```python
from build123d import *

# Parameters (mm, degrees)
F0_R     = 15.920661
F1_DEPTH = 25.4
F2_DEPTH = 65.786
F3_DEPTH = 76.2
F4_DEPTH = 61.214


with BuildPart() as f1:
    # F0 (on Top) → F1 (new body)
    with BuildSketch(Plane.XY):
        with Locations((46.579406, 0)):
            Circle(F0_R)
        with BuildLine():
            Line((46.842293, 28.102132), (-46.308367, 28.973528))
            ThreePointArc((-46.308367, 28.973528), (-17.604609, 0), (-46.308367, -28.973528))
            Line((-46.308367, -28.973528), (46.842293, -28.102132))
            ThreePointArc((46.842293, -28.102132), (74.682768, 0), (46.842293, 28.102132))
        make_face()
        with Locations((46.579406, 0)):
            Circle(F0_R, mode=Mode.SUBTRACT)
        with BuildLine():
            ThreePointArc((-46.308367, -28.973528), (-17.604609, 0), (-46.308367, 28.973528))
            ThreePointArc((-46.308367, 28.973528), (-75.554202, 0), (-46.308367, -28.973528))
        make_face()
        with Locations((-46.579406, 0)):
            Circle(F0_R, mode=Mode.SUBTRACT)
        with Locations((-46.579406, 0)):
            Circle(F0_R)
    extrude(amount=F1_DEPTH)

    # F0 (on Top) → F2 (join)
    with BuildSketch(Plane.XY):
        with BuildLine():
            ThreePointArc((-46.308367, -28.973528), (-17.604609, 0), (-46.308367, 28.973528))
            ThreePointArc((-46.308367, 28.973528), (-75.554202, 0), (-46.308367, -28.973528))
        make_face()
        with Locations((-46.579406, 0)):
            Circle(F0_R, mode=Mode.SUBTRACT)
        with Locations((-46.579406, 0)):
            Circle(F0_R)
    extrude(amount=F2_DEPTH)

    # F0 (on Top) → F3 (cut)
    with BuildSketch(Plane.XY):
        with Locations((-46.579406, 0)):
            Circle(F0_R)
    extrude(amount=F3_DEPTH, mode=Mode.SUBTRACT)

    # F0 (on Top) → F4 (cut)
    with BuildSketch(Plane.XY):
        with Locations((46.579406, 0)):
            Circle(F0_R)
    extrude(amount=F4_DEPTH, mode=Mode.SUBTRACT)


solid = f1.part
```
Could you check a few things on this model? Use its own coordinates, in mm. Coordinates: 2 decimals unless noted, no trailing zeros. Write each loop counter-clockwise with the first axis right and the second up, starting at its lowest first coordinate (ties: lowest second). Pieces come first, ordered by that corner, then holes. Notation, with made-up numbers: (14.25, 72) -> (55.25, 72) arc R15 ccw to (55.25, 80) -> close; hole circle Ø4 at (-10, 46.5). An arc over 180 degrees is marked (long way). One line per question, with ' | ' between items. Start each with the question number.
1. If we section it at B-B (x = 34.5): Please give me the cut outline in (y, z), and give its area (3 significant figures).
2. If we section it at D-D (y = 9.5): Please give me the cut outline in (x, z), and give its area (3 significant figures).
3. If we section it at C-C (y = 0): Please give me the cut outline in (x, z), and give its area (3 significant figures).
4. Will these pins go through, and if not, where does the flat tip stop? P1, Ø1, axis at x = -52.5, z = 30.5, coming from the +Y side; P2, Ø5, axis at x = -20, z = 54.5, coming from the +Y side; P3, Ø17.5, axis at x = 3.5, y = 13.5, coming from the +Z side.
5. Please list where these lines run through material, in increasing order: line 1 along X through (y, z) = (10.5, 10); line 2 along X through (y, z) = (7, 18); line 3 along X through (y, z) = (0, 45.5).
6. If we section it at A-A (z = 4.5): Please give me the cut outline in (x, y).
7. Thinking about a two-plate mould opening in X: for faces 1 (the face through (74.676, -0.614, 12.522)), 2 (the face through (61.765, 4.782, 12.522)), 3 (the face through (-59.21, -9.69, 32.43)), 4 (the face through (13, 0, 25.4)), which applies, pulls with the +X half, pulls with the -X half, needs draft (parallel to the pull), parting line crosses it, or undercut?
Return value:
1) outline: (-28.22, 0) -> (-10.37, 0) -> (-10.37, 25.4) -> (-28.22, 25.4) -> close; (10.37, 0) -> (28.22, 0) -> (28.22, 25.4) -> (10.37, 25.4) -> close | area: 907 mm²
2) outline: (-73.95, 0) -> (-59.36, 0) -> (-59.36, 65.79) -> (-73.95, 65.79) -> close; (-33.8, 0) -> (33.8, 0) -> (33.8, 25.4) -> (-19.21, 25.4) -> (-19.21, 65.79) -> (-33.8, 65.79) -> close; (59.36, 0) -> (73.03, 0) -> (73.03, 25.4) -> (59.36, 25.4) -> close | area: 3,610 mm²
3) outline: (-75.55, 0) -> (-62.5, 0) -> (-62.5, 65.79) -> (-75.55, 65.79) -> close; (-30.66, 0) -> (30.66, 0) -> (30.66, 25.4) -> (-17.6, 25.4) -> (-17.6, 65.79) -> (-30.66, 65.79) -> close; (62.5, 0) -> (74.68, 0) -> (74.68, 25.4) -> (62.5, 25.4) -> close | area: 3,250 mm²
4) P1: stops at y = 28.46 | P2: stops at y = 16.12 | P3: stops at z = 25.4
5) line 1: x = -73.58 to -58.55, -34.61 to 34.61, 58.55 to 72.65 | line 2: x = -74.7 to -60.88, -32.28 to 32.28, 60.88 to 73.8 | line 3: x = -75.55 to -62.5, -30.66 to -17.6
6) outline: (-46.31, -28.97) -> (46.84, -28.1) arc R28.1 ccw to (46.84, 28.1) -> (-46.31, 28.97) arc R28.97 ccw (long way) to start; hole circle Ø31.84 at (-46.58, 0); hole circle Ø31.84 at (46.58, 0)
7) face 1: pulls with the +X half | face 2: undercut | face 3: undercut | face 4: needs draft
